The model under review builds one solid part; all positions refer to its coordinate system, in mm. Face numbers are marked on the shaded views. A direction names the side the tool comes from. Give positions to 0.01 mm unless a question says otherwise; leave off trailing zeros. Write each loop counter-clockwise with the first axis right and the second up, starting at its lowest first coordinate (ties: lowest second). Pieces come first, ordered by that corner, then holes. Notation, with made-up numbers: (52.25, 52.5) - (59.25, 52.5) arc R20 cw to (59.25, 88.5) - close; hole circle Ø1 at (50, 19.5). An arc over 180 degrees is marked (long way). Write item = value, one per line.
```python
from build123d import *

# Parameters (mm, degrees)
SKETCH2_W                = 311.404
SKETCH2_H                = 311.404
BOSS_EXTRUDE1_DEPTH      = 67.31
SKETCH4_W                = 289.56
SKETCH4_H                = 289.56
CUT_EXTRUDE1_DEPTH       = 25.4
SKETCH5_W                = 273.304
SKETCH5_H                = 273.304
CUT_EXTRUDE2_DEPTH       = 60.96
SKETCH6_W                = 304.8
SKETCH6_H                = 304.8
SKETCH6_W_2              = 298.196
SKETCH6_H_2              = 298.196
CUT_EXTRUDE3_DEPTH       = 12.7
CUT_EXTRUDE4_REACH       = 356.607
CUT_EXTRUDE5_DEPTH       = 17.45
CUT_EXTRUDE6_REACH       = 356.607
SKETCH11_W               = 76.2
SKETCH11_H               = 20.32
CUT_EXTRUDE7_DEPTH       = 17.45
CUT_EXTRUDE8_DEPTH       = 354.20286992
CUT_EXTRUDE8_DEPTH_BACK  = 354.20286992
SKETCH12_OUTSIDE_W       = 402.506
SKETCH12_OUTSIDE_H       = 158.412
SKETCH13_W               = 110.05
SKETCH13_H               = 51.5
SKETCH13_W_2             = 97.35
SKETCH13_H_2             = 38.8
BOSS_EXTRUDE2_DEPTH      = 1.6
BOSS_EXTRUDE3_DEPTH      = 38.1
BOSS_EXTRUDE3_DEPTH_BACK = 1.6
SKETCH15_W               = 110.05
SKETCH15_H               = 3
RIB1_REACH               = 199.5
SKETCH16_WALL_W          = 461.061960636
SKETCH16_WALL_H          = 2.54


with BuildPart() as part:
    # Sketch2 → Boss-Extrude1 (new body)
    with BuildSketch(Plane(origin=(0, 0, 0), x_dir=(1, 0, 0), z_dir=(0, 1, 0))):
        Rectangle(SKETCH2_W, SKETCH2_H)
    extrude(amount=BOSS_EXTRUDE1_DEPTH)

    # Sketch4 → Cut-Extrude1 (cut)
    with BuildSketch(Plane(origin=(0, 67.31, 0), x_dir=(1, 0, 0), z_dir=(0, 1, 0))):
        Rectangle(SKETCH4_W, SKETCH4_H)
    extrude(amount=-CUT_EXTRUDE1_DEPTH, mode=Mode.SUBTRACT)

    # Sketch5 → Cut-Extrude2 (cut)
    with BuildSketch(Plane(origin=(0, 67.31, 0), x_dir=(1, 0, 0), z_dir=(0, 1, 0))):
        Rectangle(SKETCH5_W, SKETCH5_H)
    extrude(amount=-CUT_EXTRUDE2_DEPTH, mode=Mode.SUBTRACT)

    # Sketch6 → Cut-Extrude3 (cut)
    with BuildSketch(Plane(origin=(0, 67.31, 0), x_dir=(1, 0, 0), z_dir=(0, 1, 0))):
        Rectangle(SKETCH6_W, SKETCH6_H)
        Rectangle(SKETCH6_W_2, SKETCH6_H_2, mode=Mode.SUBTRACT)
    extrude(amount=-CUT_EXTRUDE3_DEPTH, mode=Mode.SUBTRACT)

    # Sketch7 → Cut-Extrude4 (cut, up to next)
    with BuildSketch(Plane.ZY.offset(155.702), mode=Mode.PRIVATE) as cut_extrude4_sk1:
        with BuildLine():
            Line((-29.275, 43.15), (29.275, 43.15))
            ThreePointArc((29.275, 43.15), (46.675, 25.75), (29.275, 8.35))
            Line((29.275, 8.35), (-29.275, 8.35))
            ThreePointArc((-29.275, 8.35), (-46.675, 25.75), (-29.275, 43.15))
        make_face()
    cut_extrude4_tool1 = extrude(cut_extrude4_sk1.sketch, amount=-CUT_EXTRUDE4_REACH, mode=Mode.PRIVATE) & part.part
    add(cut_extrude4_tool1.solids().sort_by_distance((-155.702, 25.75, 0))[0], mode=Mode.SUBTRACT)

    # Sketch8 → Cut-Extrude5 (cut)
    with BuildSketch(Plane(origin=(-136.652, 0, 0), x_dir=(0, 0, -1), z_dir=(1, 0, 0))):
        Polygon((29.275, 45.15), (48.675, 45.15), (48.675, 25.75), (48.675, 6.35), (29.275, 6.35), (-29.275, 6.35), (-48.675, 6.35), (-48.675, 25.75), (-48.675, 45.15), (-29.275, 45.15), align=None)
    extrude(amount=-CUT_EXTRUDE5_DEPTH, mode=Mode.SUBTRACT)

    # Sketch9 → Cut-Extrude6 (cut, up to next)
    with BuildSketch(Plane.ZY.offset(155.702), mode=Mode.PRIVATE) as cut_extrude6_sk1:
        with BuildLine():
            Line((46.014100932, 30.5), (48.175, 30.5))
            Line((48.175, 30.5), (48.175, 21))
            Line((48.175, 21), (46.014100932, 21))
            ThreePointArc((46.014100932, 21), (46.675, 25.75), (46.014100932, 30.5))
        make_face()
    cut_extrude6_tool1 = extrude(cut_extrude6_sk1.sketch, amount=-CUT_EXTRUDE6_REACH, mode=Mode.PRIVATE) & part.part
    add(cut_extrude6_tool1.solids().sort_by_distance((-155.702, 25.75, 47.304468))[0], mode=Mode.SUBTRACT)

    # Sketch11 → Cut-Extrude7 (cut)
    with BuildSketch(Plane(origin=(-136.652, 0, 0), x_dir=(0, 0, -1), z_dir=(1, 0, 0))):
        with Locations((-86.775, 25.4)):
            Rectangle(SKETCH11_W, SKETCH11_H)
    extrude(amount=-CUT_EXTRUDE7_DEPTH, mode=Mode.SUBTRACT)

    # Sketch12 outside → Cut-Extrude8 (cut, two sides: drawn at the far end of the back side and taken through both)
    with BuildSketch(Plane(origin=(-154.102, 0, 0), x_dir=(0, 0, -1), z_dir=(1, 0, 0)).offset(-CUT_EXTRUDE8_DEPTH_BACK)):
        with Locations((0, 33.655)):
            Rectangle(SKETCH12_OUTSIDE_W, SKETCH12_OUTSIDE_H)
        Polygon((-48.675, 35.56), (-48.675, 15.24), (-48.675, 6.35), (48.675, 6.35), (48.675, 45.15), (-48.675, 45.15), align=None, mode=Mode.SUBTRACT)
    extrude(amount=CUT_EXTRUDE8_DEPTH + CUT_EXTRUDE8_DEPTH_BACK, mode=Mode.SUBTRACT)


with BuildPart() as cut_extrude8_kept_piece:
    # of the separate pieces the step leaves, the one the design keeps (cut_extrude8_pieces_kept)
    add(part.part.solids().sort_by_distance((-155.702, 6.35, 48.675))[0])

    # Sketch13 → Boss-Extrude2 (add)
    with BuildSketch(Plane(origin=(-154.102, 0, 0), x_dir=(0, 0, -1), z_dir=(1, 0, 0))):
        with Locations((0, 25.75)):
            Rectangle(SKETCH13_W, SKETCH13_H)
        with Locations((0, 25.75)):
            Rectangle(SKETCH13_W_2, SKETCH13_H_2, mode=Mode.SUBTRACT)
    extrude(amount=-BOSS_EXTRUDE2_DEPTH)

    # Sketch15 → Boss-Extrude3 (add, two sides: drawn at the far end of the back side and taken through both)
    with BuildSketch(Plane(origin=(-154.102, 0, 0), x_dir=(0, 0, -1), z_dir=(1, 0, 0)).offset(-BOSS_EXTRUDE3_DEPTH_BACK)):
        with Locations((0, -1.5)):
            Rectangle(SKETCH15_W, SKETCH15_H)
    extrude(amount=BOSS_EXTRUDE3_DEPTH + BOSS_EXTRUDE3_DEPTH_BACK)

    # Sketch16 wall → Rib1 (add, up to next)
    with BuildSketch(Plane(origin=(-135.052, 25.75, 55.025), x_dir=(0.594742134678, -0.803916533751, 0), z_dir=(0.803916533751, 0.594742134678, 0)), mode=Mode.PRIVATE) as rib1_sk1:
        with Locations((0, 1.27)):
            Rectangle(SKETCH16_WALL_W, SKETCH16_WALL_H)
    rib1_tool1 = extrude(rib1_sk1.sketch, amount=-RIB1_REACH, mode=Mode.PRIVATE) - cut_extrude8_kept_piece.part
    rib1 = rib1_tool1.solids().sort_by_distance((-135.052, 25.75, 55.025))[0]
    add(rib1)

    # Mirror1: Rib1 across plane
    add(rib1.mirror(Plane.XY))


solid = cut_extrude8_kept_piece.part
```
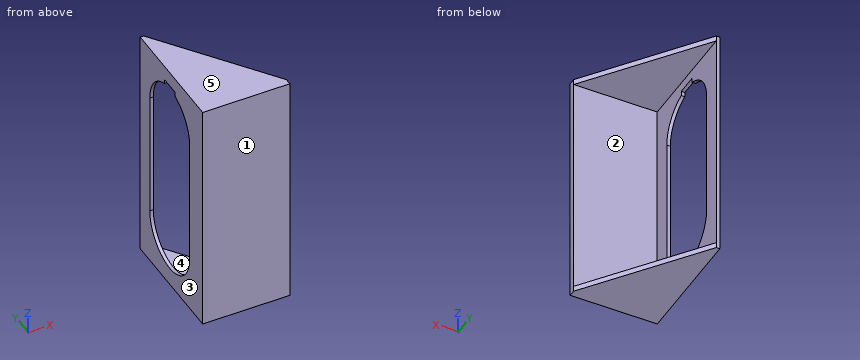
1. Take a section at C-C on x = -122.5. Give the boundary of the cut face in (y, z) (3 decimals), and give its area (3 significant figures).
Findings below:
outline = (-3, -55.025) - (8.783, -55.025) - (8.783, -52.485) - (0, -52.485) - (0, 52.485) - (8.783, 52.485) - (8.783, 55.025) - (-3, 55.025) - close
area = 375 mm²
2. Machinability: for the marked faces 1 and 2, which of the approach directions +Z, -Z, +X, -X, +Y, -Y give a long, thin tool a straight path to every point of the face, cutting with its end or side? Answer none if there is none.
Findings below:
face_1 = +Z, -Z, +X, -X, -Y
face_2 = +X, +Y
3. Take a section at A-A on z = 20. Give the boundary of the cut face in (x, y), and give its area (3 significant figures).
Findings below:
outline = (-155.7, -3) - (-116, -3) - (-116, 0) - (-154.1, 0) - (-154.1, 8.35) - (-155.7, 8.35) - close; (-155.7, 43.15) - (-154.1, 43.15) - (-154.1, 51.5) - (-155.7, 51.5) - close
area = 146 mm²
4. Take a section at D-D on y = 10. Give the boundary of the cut face in (x, z) (3 decimals).
Findings below:
outline = (-155.702, -55.025) - (-123.4, -55.025) - (-123.4, -52.485) - (-154.102, -52.485) - (-154.102, -36.671) - (-155.702, -36.671) - close; (-155.702, 36.671) - (-154.102, 36.671) - (-154.102, 52.485) - (-123.4, 52.485) - (-123.4, 55.025) - (-155.702, 55.025) - close
5. Take a section at B-B on y = 25.75. Give the boundary of the cut face in (x, z) (3 decimals).
Findings below:
outline = (-155.702, -55.025) - (-135.052, -55.025) - (-135.052, -52.485) - (-154.102, -52.485) - (-154.102, -46.675) - (-155.702, -46.675) - close; (-155.702, 48.175) - (-154.102, 48.175) - (-154.102, 52.485) - (-135.052, 52.485) - (-135.052, 55.025) - (-155.702, 55.025) - close
6. For line 1 (Z direction, x = -152, y = 2) (3 decimals); line 2 (Y direction, x = -148, z = -9.5); line 3 (X direction, y = 1, z = -23), list the stretches that pass through material, from the lowest coordinate up. Write a range as from..to.
Findings below:
line_1 = -55.025..-52.485, 52.485..55.025
line_2 = -3..0
line_3 = -155.7..-154.1
7. Insertion check: P1, Ø11.5, axis at x = -140.5, y = 35, coming from the +Z side (3 decimals); P2, Ø15.5, axis at y = 36, z = 23, coming from the +X side. Each pin has a flat end and moves straight along its axis. Give the tip position at first contact, or say it passes through.
Findings below:
P1 = 55.025
P2 = -154.1
8. Draft analysis for pull direction Z (two halves, no side actions). For the marked faces 3, 4 and 5, state which applies: +Z half, -Z half, draft (parallel to the pull), parting line (faces both ways), or undercut.
Findings below:
face_3 = draft
face_4 = undercut
face_5 = +Z half
